The figure shows three views and two pictorial views of one solid part (mm, origin at its lowest corner). Answer the questions. A direction names the side the tool comes from. Give positions to 0.01 mm unless a question says otherwise; leave off trailing zeros. Order: outer loops, then holes, each group sorted by start corner. A loop starts at its lowest first (then second) coordinate and runs counter-clockwise, first axis right, second up. Notation, with made-up numbers: (-21, 89) - (4, 89) arc R15 cw to (4, 110) - close; hole circle Ø11 at (40.25, -20). An arc over 180 degrees is marked (long way). Answer as CSV lines item,"result". Start each with the question number.
1. Flat-ended cylindrical pins translate along their axes: pin 1 (2 mm diameter, centred on x = 3.5, z = 10, fed in from +Y); pin 2 (6 mm diameter, centred on y = 10, z = 11.5, fed in from +X); pin 3 (10 mm diameter, centred on x = 23.5, z = 11, fed in from +Y). Find the tip coordinate at first contact, or state that the pin passes through.
2. Consider line 1 along X through (y, z) = (23, 12.75); line 2 along Y through (x, z) = (10, 2); line 3 along Y through (x, z) = (53, 5.25). Determine where each line is inside the solid, lowest interval first. Write a range as [from, to].
3. Section A-A on z = 18.5 is taken. Give the vertices of the cut face in (x, y), and give its area (3 significant figures).
4. Section D-D on z = 8.75 is taken. Give the vertices of the cut face in (x, y).
5. Section B-B on x = 37.6 is taken. Give the vertices of the cut face in (y, z), and give its area (3 significant figures).
6. Which of the six approach directions +Z, -Z, +X, -X, +Y, -Y give full straight-line access (tool end or side, diameter ignored) to the marked faces 1, 2 and 3?
7. Section C-C on y = 14.5 is taken. Give the vertices of the cut face in (x, z).
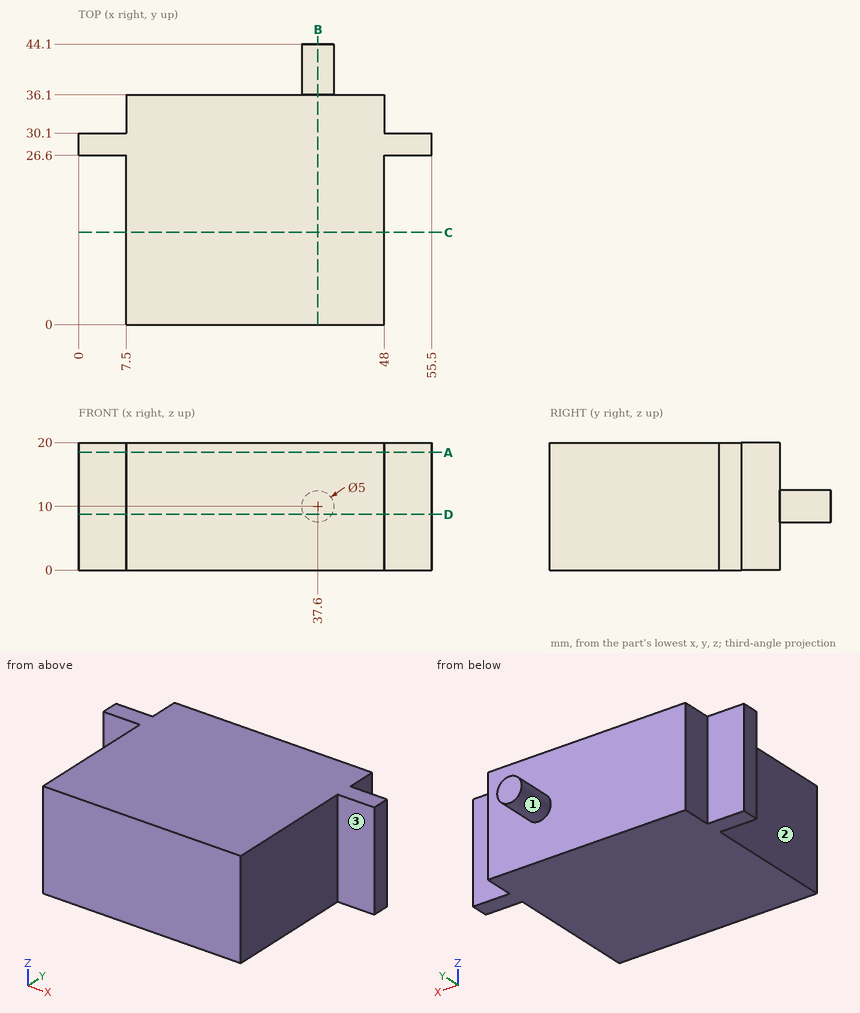
Checks:
1,pin 1,"stops at y = 30.1"
1,pin 2,"stops at x = 48"
1,pin 3,"stops at y = 36.1"
2,line 1,"x = [7.5, 48]"
2,line 2,"y = [0, 36.1]"
2,line 3,"y = [26.6, 30.1]"
3,outline,"(0, 26.6) - (7.5, 26.6) - (7.5, 0) - (48, 0) - (48, 26.6) - (55.5, 26.6) - (55.5, 30.1) - (48, 30.1) - (48, 36.1) - (7.5, 36.1) - (7.5, 30.1) - (0, 30.1) - close"
3,area,"1,510 mm²"
4,outline,"(0, 26.6) - (7.5, 26.6) - (7.5, 0) - (48, 0) - (48, 26.6) - (55.5, 26.6) - (55.5, 30.1) - (48, 30.1) - (48, 36.1) - (39.77, 36.1) - (39.77, 44.1) - (35.43, 44.1) - (35.43, 36.1) - (7.5, 36.1) - (7.5, 30.1) - (0, 30.1) - close"
5,outline,"(0, 0) - (36.1, 0) - (36.1, 7.5) - (44.1, 7.5) - (44.1, 12.5) - (36.1, 12.5) - (36.1, 20) - (0, 20) - close"
5,area,"762 mm²"
6,face 1,"+Y"
6,face 2,"+Z, -Z, -X, -Y"
6,face 3,"+Z, -Z, +X, -Y"
7,outline,"(7.5, 0) - (48, 0) - (48, 20) - (7.5, 20) - close"
